The listing builds one solid part. Answer for the finished solid, in the listing's coordinates (mm). Coordinates: 2 decimals unless noted, no trailing zeros. Write each loop counter-clockwise with the first axis right and the second up, starting at its lowest first coordinate (ties: lowest second). Pieces come first, ordered by that corner, then holes. Notation, with made-up numbers: M 19,-4 L 34,-4 A23 ccw 34,7 Z; hole C 41.5,2.25 d5. An arc over 180 degrees is marked long. Answer as CSV lines item,"result".
```python
from build123d import *

# Parameters (mm, degrees)
SKETCH1_W           = 152.4
SKETCH1_H           = 44.45
BOSS_EXTRUDE1_DEPTH = 6.35
SKETCH2_W           = 146.05
SKETCH2_H           = 6.35
CUT_EXTRUDE1_DEPTH  = 1.6002
SKETCH3_R           = 1.18745
CUT_EXTRUDE2_DEPTH  = 5.7498
SKETCH4_W           = 6.35
SKETCH4_H           = 6.35
CUT_EXTRUDE3_DEPTH  = 1.6002


with BuildPart() as part:
    # Sketch1 → Boss-Extrude1 (new body)
    with BuildSketch(Plane(origin=(0, 0, 0), x_dir=(1, 0, 0), z_dir=(0, 1, 0))):
        with Locations((76.2, 22.225)):
            Rectangle(SKETCH1_W, SKETCH1_H)
    extrude(amount=BOSS_EXTRUDE1_DEPTH)

    # Sketch2 → Cut-Extrude1 (cut)
    with BuildSketch(Plane(origin=(0, 6.35, 0), x_dir=(1, 0, 0), z_dir=(0, 1, 0))):
        with Locations((73.025, 34.925)):
            Rectangle(SKETCH2_W, SKETCH2_H)
    extrude(amount=-CUT_EXTRUDE1_DEPTH, mode=Mode.SUBTRACT)

    # Sketch3 → Cut-Extrude2 (cut, through all)
    with BuildSketch(Plane(origin=(0, 4.7498, 0), x_dir=(1, 0, 0), z_dir=(0, 1, 0))):
        with Locations((25.4, 34.925)):
            Circle(SKETCH3_R)
    extrude(amount=-CUT_EXTRUDE2_DEPTH, mode=Mode.SUBTRACT)

    # Sketch4 → Cut-Extrude3 (cut)
    with BuildSketch(Plane(origin=(0, 6.35, 0), x_dir=(1, 0, 0), z_dir=(0, 1, 0))):
        with Locations((149.225, 34.925)):
            Rectangle(SKETCH4_W, SKETCH4_H)
    extrude(amount=-CUT_EXTRUDE3_DEPTH, mode=Mode.SUBTRACT)


solid = part.part
```
Q1. A flat-ended cylindrical pin translates along its axis: pin 1 Ø1.9 at (x, z) = (51, -36) entering from +Y. Find the tip coordinate at first contact, or state that the pin passes through.
Output:
pin 1,"y = 4.75"
Q2. Find section A-A (x = 81). Give the vertices of the cut face in (y, z), and give its area (3 significant figures).
Output:
outline,"M 0,-44.45 L 6.35,-44.45 L 6.35,-38.1 L 4.75,-38.1 L 4.75,-31.75 L 6.35,-31.75 L 6.35,0 L 0,0 Z"
area,"272 mm2"
Q3. Straight lines are drawn through the part: line 1 (Z direction, x = 25.4, y = 2.45); line 2 (Z direction, x = 72, y = 5.25); line 3 (Y direction, x = 83, z = -36.5). For each, find the intervals that lie inside material, in ascending order.
Output:
line 1,"-44.45 to -36.11, -33.74 to 0"
line 2,"-44.45 to -38.1, -31.75 to 0"
line 3,"0 to 4.75"
Q4. The mould has two halves that part along Z. Classify faces 1 (the flat face through (75, 3, 0)), 2 (the flat face through (75, 6.35, -16)), 3 (the flat face through (75, 4.75, -35)): pulls with the +Z half, pulls with the -Z half, needs draft (parallel to the pull), parting line crosses it, or undercut.
Output:
face 1,"pulls with the +Z half"
face 2,"needs draft"
face 3,"undercut"
